Design review of the part built by this model. Coordinates are the model's own, in mm. A direction names the side the tool comes from. Coordinates: 2 decimals unless noted, no trailing zeros. Loops run counter-clockwise (first coordinate to the right, second up) from the corner with the lowest first, then second, coordinate; pieces in that order, holes last.
Q1. Machinability: for faces 4 (the face through (47.25, -5.51, -47.04)), 5 (the face through (24.9, -23.45, 5.02)), which of the approach directions +Z, -Z, +X, -X, +Y, -Y give a long, thin tool a straight path to every point of the face, cutting with its end or side? Answer none if there is none.
Q2. Add section A-A on y = -9. Give the number of separate pieces and of enclosed holes in the cut face, and give its area (3 significant figures).
Q3. Wall thickness on probe 1 along X at (y, z) = (-6, -54); probe 2 along X at (y, z) = (-2, -50); probe 3 along Y at (x, z) = (16, -52): over which ranges is each line inside the solid? List them lowest first.
Q4. Draft analysis for pull direction Z (two halves, no side actions). For faces 1 (the face through (0, -6, -69.85)), 2 (the face through (-34.571, -5.51, -16.306)), 3 (the face through (-22.52, -5.51, -48.89)), state which applies: released by +Z, released by -Z, zero draft, split by the parting line, or undercut.
Q5. Add section B-B on y = -16. Give the boundary of the cut face in (x, z) (1 decimal).
Q6. Add section C-C on x = 40. Give the boundary of the cut face in (y, z).
Q7. For P1, Ø3, axis at y = -10.5, z = -6, coming from the -X side; P2, Ø1.5, axis at y = -18.5, z = 11.5, coming from the +X side; P3, Ø6, axis at y = -36, z = 10, coming from the -X side, all flat-tipped, find the tip position at first contact; note any pin that passes through.
```python
from build123d import *

# Parameters (mm, degrees)
F0_R     = 14.2875
F1_DEPTH = 41.148
F2_R     = 5.08
F3_DEPTH = 11.176
F0_R_2   = 6.35
F4_DEPTH = 11.176
F5_DEPTH = 11.176


with BuildPart() as f1:
    # F0 (on Front) → F1 (new body)
    with BuildSketch(Plane.XZ):
        with BuildLine():
            ThreePointArc((-23.36292, 9.966643), (-5.086346, -24.88552), (25.4, 0))
            ThreePointArc((25.4, 0), (24.88552, 5.086346), (23.36292, 9.966643))
            ThreePointArc((23.36292, 9.966643), (0, 25.4), (-23.36292, 9.966643))
        make_face()
        Circle(F0_R, mode=Mode.SUBTRACT)
    extrude(amount=F1_DEPTH)

    # F2
    f2_edges = [f1.edges().sort_by_distance(p)[0] for p in [
        (-25.4, -41.148, 0),
        (-14.2875, -41.148, 0),
    ]]
    fillet(f2_edges, radius=F2_R)

    # F0 (on Front) → F3 (join)
    with BuildSketch(Plane.XZ):
        with BuildLine():
            ThreePointArc((23.36292, 9.966643), (24.88552, 5.086346), (25.4, 0))
            ThreePointArc((25.4, 0), (-5.086346, -24.88552), (-23.36292, 9.966643))
            Line((-23.36292, 9.966643), (-46.09719, -43.325018))
            ThreePointArc((-46.09719, -43.325018), (-24.760241, -32.13586), (-9.525, -50.8))
            ThreePointArc((-9.525, -50.8), (-15.104616, -64.270384), (-28.575, -69.85))
            Line((-28.575, -69.85), (28.575, -69.85))
            ThreePointArc((28.575, -69.85), (12.680018, -40.299903), (46.09719, -43.325018))
            Line((46.09719, -43.325018), (23.36292, 9.966643))
        make_face()
    extrude(amount=F3_DEPTH)

    # F0 (on Front) → F4 (join)
    with BuildSketch(Plane.XZ):
        with BuildLine():
            ThreePointArc((-9.525, -50.8), (-24.760241, -32.13586), (-46.09719, -43.325018))
            ThreePointArc((-46.09719, -43.325018), (-44.469982, -61.300097), (-28.575, -69.85))
            ThreePointArc((-28.575, -69.85), (-15.104616, -64.270384), (-9.525, -50.8))
        make_face()
        with Locations((-28.575, -50.8)):
            Circle(F0_R_2, mode=Mode.SUBTRACT)
    extrude(amount=F4_DEPTH)

    # F0 (on Front) → F5 (join)
    with BuildSketch(Plane.XZ):
        with BuildLine():
            ThreePointArc((47.625, -50.8), (47.23914, -46.985241), (46.09719, -43.325018))
            ThreePointArc((46.09719, -43.325018), (12.680018, -40.299903), (28.575, -69.85))
            ThreePointArc((28.575, -69.85), (42.045384, -64.270384), (47.625, -50.8))
        make_face()
        with Locations((28.575, -50.8)):
            Circle(F0_R_2, mode=Mode.SUBTRACT)
    extrude(amount=F5_DEPTH)


solid = f1.part
```
Entries:
1. face 4: +Z, +X, +Y, -Y
1. face 5: +Z, +X, -Y
2. separate pieces: 1
2. enclosed holes: 3
2. area: 5,690 mm2
3. probe 1: x = -47.35 to -34.06, -23.09 to 23.09, 34.06 to 47.35
3. probe 2: x = -47.61 to -34.87, -22.28 to 22.28, 34.87 to 47.61
3. probe 3: y = -11.18 to 0
4. face 1: released by -Z
4. face 2: released by +Z
4. face 3: undercut
5. outline: (23.4, 10) arc R25.4 ccw (long way) to (25.4, 0) arc R25.4 ccw to start; hole circle Ø28.6 at (0, 0)
6. outline: (-11.18, -66.04) - (0, -66.04) - (0, -29.03) - (-11.18, -29.03) - close
7. P1: stops at x = -30.81
7. P2: stops at x = 23.01
7. P3: stops at x = -24.42
